Could you check a few things on this model? Use its own coordinates, in mm. Face numbers are marked on the shaded views. A direction names the side the tool comes from. Coordinates: 2 decimals unless noted, no trailing zeros. Loops run counter-clockwise (first coordinate to the right, second up) from the corner with the lowest first, then second, coordinate; pieces in that order, holes last. Notation, with made-up numbers: (12, -37.5) - (37, -37.5) arc R26 ccw to (37, -17.5) - close; hole circle Ø8 at (51, 30.5). An arc over 180 degrees is marked (long way). One line per item, written item: value. Start each with the question number.
(1) If we section it at D-D on y = 12: Write out the boundary of the cut face in (x, z).
(2) I'm going to push flat-ended pins straight in: P1, Ø4, axis at y = 26, z = 4.5, coming from the -X side; P2, Ø1, axis at x = 0, z = -13, coming from the +Y side; P3, Ø2, axis at y = 16, z = 1.5, coming from the +X side. Where does each tip first touch, or does it pass through?
(3) If we section it at B-B on z = 0: Write out the boundary of the cut face in (x, y), then the cut area to 3 significant figures.
(4) If we section it at C-C on x = -22: Write out the boundary of the cut face in (y, z).
(5) If we section it at A-A on y = 7: Write out the boundary of the cut face in (x, z).
(6) On a 3-axis mill with a long thin cutter (end or side, diameter ignored), from which of +Z, -Z, +X, -X, +Y, -Y can I reach the whole of each face in a straight line? I mean the marked faces 1, 2, 3 and 4. Say none if no direction works.
(7) If we mould it in two halves opening along Z, with no side actions, what happens to the marked faces 5, 6, 7 and 8? For each: pulls with the +Z half, pulls with the -Z half, needs draft (parallel to the pull), parting line crosses it, or undercut.
(8) If I drill on line 1 along Y through (x, z) = (-20, -4.25); line 2 along Y through (x, z) = (-12.5, 12.75); line 3 along X through (y, z) = (8.5, 5.75), over which ranges is the centre line in solid material (lowest first)? Write a range as from..to.
Autodesk Inventor part; units mm, degrees
ref_plane "Work Plane1" through (0, 33, 0) normal (0, 1, 0) x (-1, 0, 0)
ref_plane "YZ Plane" through (0, 0, 0) normal (1, 0, 0) x (0, 1, 0)
ref_plane "XY Plane" through (0, 0, 0) normal (0, 0, 1) x (1, 0, 0)
ref_plane "Work Plane1" through (0, 33, 0) normal (0, 1, 0) x (-1, 0, 0)
sketch "Sketch1" plane through (0, 33, 0) normal (0, 1, 0) x (-1, 0, 0)
  line L0 (-27.5, 15) -> (-27.5, -15)
  line L1 (-27.5, 15) -> (27.5, 15)
  line L2 (27.5, 15) -> (27.5, -15)
  line L3 (-27.5, -15) -> (27.5, -15)
extrude "Extrusion13" add sketch "Sketch1" against normal blind 33
sketch "Sketch2" plane through (-27.5, 33, 15) normal (0, 0, 1) x (1, 0, 0)
  line L0 (18.25, -25) -> (12.75, -25)
  line L1 (12.75, -29) -> (18.25, -29)
  line L2 (18.25, -29) -> (18.25, -25)
  line L3 (12.75, -25) -> (12.75, -29)
extrude "Extrusion12" cut sketch "Sketch2" against normal blind 30
sketch "Sketch3" plane through (-14.75, 4, 15) normal (0, 1, 0) x (1, 0, 0)
  arc A0 (1.5126, 6.7374) -> (3.9874, 6.7374) centre (2.75, 5.5) ccw
  line L0 (3.9874, 6.7374) -> (2.75, 7.9749)
  line L1 (2.75, 7.9749) -> (1.5126, 6.7374)
extrude "Extrusion11" cut sketch "Sketch3" against normal blind 4
sketch "Sketch4" plane through (0, 0, 0) normal (0, 1, 0) x (-1, 0, 0)
  arc A0 (13.2374, -10.7374) -> (10.7626, -10.7374) centre (12, -9.5) ccw
  line L0 (13.2374, -10.7374) -> (12, -11.9749)
  line L1 (12, -11.9749) -> (10.7626, -10.7374)
extrude "Extrusion10" cut sketch "Sketch4" along normal blind 4
sketch "Sketch5" plane through (-14.75, 8, 15) normal (0, -1, 0) x (1, 0, 0)
  line L0 (2.75, -7.9749) -> (3.9874, -6.7374)
  line L1 (1.5126, -6.7374) -> (2.75, -7.9749)
  arc A0 (3.9874, -6.7374) -> (1.5126, -6.7374) centre (2.75, -5.5) ccw
extrude "Extrusion9" cut sketch "Sketch5" against normal blind 12
sketch "Sketch6" plane through (-14.75, 8, 15) normal (0, -1, 0) x (1, 0, 0)
  line L0 (2.75, -26.9749) -> (3.9874, -25.7374)
  line L1 (1.5126, -25.7374) -> (2.75, -26.9749)
  arc A0 (3.9874, -25.7374) -> (1.5126, -25.7374) centre (2.75, -24.5) ccw
extrude "Extrusion8" cut sketch "Sketch6" against normal blind 12
sketch "Sketch7" plane through (0, 33, 0) normal (0, 1, 0) x (-1, 0, 0)
  line L0 (-4.409, 6.0942) -> (-6, 4.5032)
  arc A0 (-4.409, 6.0942) -> (-7.591, 6.0942) centre (-6, 7.6852) ccw
  line L1 (-7.591, 6.0942) -> (-6, 4.5032)
extrude "Extrusion7" cut sketch "Sketch7" against normal blind 33
sketch "Sketch8" plane through (0, 33, 0) normal (0, 1, 0) x (-1, 0, 0)
  line L0 (-5.3033, -5.3033) -> (0, -10.6066)
  arc A0 (-3.7724, 7.3683) -> (-3.0726, 6.8417) centre (-3.2774, 7.2978) ccw
  arc A1 (-4.409, 6.0942) -> (-3.7724, 7.3683) centre (-6, 7.6852) ccw
  line L1 (0, -10.6066) -> (5.3033, -5.3033)
  arc A2 (5.3033, -5.3033) -> (-3.0726, 6.8417) centre (0, 0) ccw
  line L2 (-6, 4.5032) -> (-4.409, 6.0942)
  line L3 (-6.2969, 4.8001) -> (-6, 4.5032)
  arc A3 (-6.2348, 4.1686) -> (-6.2969, 4.8001) centre (-6.6504, 4.4466) ccw
  arc A4 (-6.2348, 4.1686) -> (-5.3033, -5.3033) centre (0, 0) ccw
extrude "Extrusion6" cut sketch "Sketch8" against normal blind 24 draft 0
sketch "Sketch9" plane through (0, 33, 0) normal (0, 1, 0) x (-1, 0, 0)
  line L0 (0, -10.6066) -> (-1, -9.6066)
  line L1 (1, -9.6066) -> (0, -10.6066)
  line L2 (-1, -9.6066) -> (-1, -15)
  line L3 (-1, -15) -> (1, -15)
  line L4 (1, -9.6066) -> (1, -15)
extrude "Extrusion5" cut sketch "Sketch9" against normal blind 23 draft 0
sketch "Sketch10" plane through (0, 33, 0) normal (0, 1, 0) x (-1, 0, 0)
  line L0 (-1, 15) -> (1, 15)
  arc A0 (1, 7.433) -> (-1, 7.433) centre (0, 0) ccw
  line L1 (-1, 15) -> (-1, 7.433)
  line L2 (1, 15) -> (1, 7.433)
extrude "Extrusion4" cut sketch "Sketch10" against normal blind 23 draft 0
sketch "Sketch11" plane through (0, 33, 0) normal (0, 1, 0) x (-1, 0, 0)
  line L0 (15, -13) -> (13, -15)
  line L1 (13, 15) -> (27.5, 15)
  line L2 (15, 13) -> (15, -13)
  line L3 (27.5, 15) -> (27.5, -15)
  line L4 (13, 15) -> (15, 13)
  line L5 (13, -15) -> (27.5, -15)
extrude "Extrusion3" cut sketch "Sketch11" against normal blind 19 draft 0
sketch "Sketch12" plane through (0, 33, 0) normal (0, 1, 0) x (-1, 0, 0)
  line L0 (-27.5, 15) -> (-13, 15)
  line L1 (-13, -15) -> (-15, -13)
  line L2 (-15, 13) -> (-13, 15)
  line L3 (-27.5, -15) -> (-13, -15)
  line L4 (-27.5, 15) -> (-27.5, -15)
  line L5 (-15, 13) -> (-15, -13)
extrude "Extrusion2" cut sketch "Sketch12" against normal blind 19 draft 0
sketch "Sketch13" plane through (0, 9, 0) normal (0, 1, 0) x (1, 0, 0)
  line L0 (0, 7.0711) -> (3.5355, 3.5355)
  arc A0 (-3.5355, 3.5355) -> (3.5355, 3.5355) centre (0, 0) ccw
  line L1 (-3.5355, 3.5355) -> (0, 7.0711)
extrude "Extrusion1" cut sketch "Sketch13" against normal blind 9
hole "Hole2" at (20, 7, 15) direction (0, 0, -1) diameter 6.5 depth 30
sketch "Sketch14" plane through (-27.5, 0, 15) normal (0, 0, 1) x (1, 0, 0)
  point P0 (47.5, 7)
hole "Hole1" at (-20, 7, 15) direction (0, 0, -1) diameter 6.5 depth 30
sketch "Sketch15" plane through (-27.5, 0, 15) normal (0, 0, 1) x (1, 0, 0)
  point P0 (7.5, 7)
properties part number "Hopper Linear Bearing Holder" material "ASA Plastic"
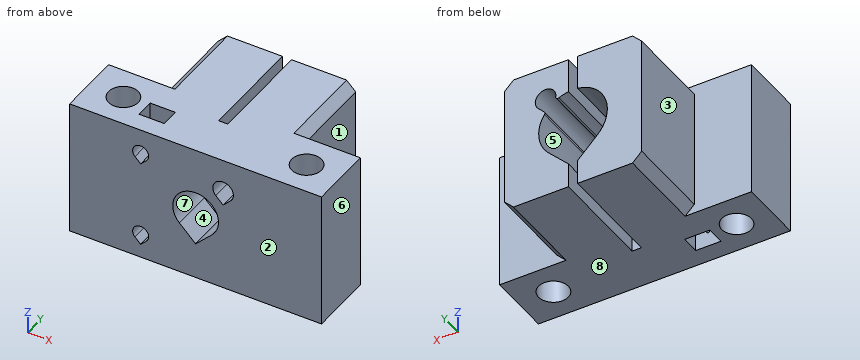
Values:
1. outline: (-27.5, -15) - (-1, -15) - (-1, -9.61) - (-5.3, -5.3) arc R7.5 cw to (-1, 7.43) - (-1, 15) - (-27.5, 15) - close; (1, -15) - (27.5, -15) - (27.5, 15) - (1, 15) - (1, 7.43) arc R7.5 cw to (3.07, 6.84) arc R0.5 ccw to (3.77, 7.37) arc R2.25 cw (long way) to (7.59, 6.09) - (6.3, 4.8) arc R0.5 ccw to (6.23, 4.17) arc R7.5 cw to (5.3, -5.3) - (1, -9.61) - close; hole (-13.24, -10.74) - (-12, -11.97) - (-10.76, -10.74) arc R1.75 ccw (long way) to start; hole (-13.24, 8.26) - (-12, 7.03) - (-10.76, 8.26) arc R1.75 ccw (long way) to start
2. P1: stops at x = -15
2. P2: stops at y = 10
2. P3: stops at x = 15
3. outline: (-27.5, 0) - (-5, 0) - (-5, 9) - (-7.5, 9) - (-7.5, 33) - (-15, 33) - (-15, 14) - (-27.5, 14) - close; (5, 0) - (27.5, 0) - (27.5, 14) - (15, 14) - (15, 33) - (7.5, 33) - (7.5, 9) - (5, 9) - close; hole circle Ø6.5 at (-20, 7); hole (-14.75, 4) - (-9.25, 4) - (-9.25, 8) - (-14.75, 8) - close; hole circle Ø6.5 at (20, 7)
3. area: 802 mm2
4. outline: (0, -15) - (4.44, -15) - (4.44, 15) - (0, 15) - close; (9.56, -15) - (14, -15) - (14, 15) - (9.56, 15) - close
5. outline: (-27.5, -15) - (-23.25, -15) - (-23.25, 15) - (-27.5, 15) - close; (-16.75, -15) - (-14.75, -15) - (-14.75, 15) - (-16.75, 15) - close; (-9.25, -15) - (16.75, -15) - (16.75, 15) - (-9.25, 15) - close; (23.25, -15) - (27.5, -15) - (27.5, 15) - (23.25, 15) - close; hole (-3.54, -3.54) - (0, -7.07) - (3.54, -3.54) arc R5 ccw (long way) to start; hole (4.41, 6.09) - (6, 4.5) - (7.59, 6.09) arc R2.25 ccw (long way) to start
6. face 1: +Z, -Z, +X, +Y
6. face 2: +Z, -Z, +X, -X, -Y
6. face 3: +Z, -Z, -X, +Y
6. face 4: +Y, -Y
7. face 5: undercut
7. face 6: needs draft
7. face 7: undercut
7. face 8: pulls with the -Z half
8. line 1: y = 0..3.75, 10.25..14
8. line 2: y = 0..4, 8..33
8. line 3: x = -27.5..-22.88, -17.12..4.75, 7.25..17.12, 22.88..27.5
